Work out the finished part from the listing and answer in its coordinate system (mm). A direction names the side the tool comes from. Coordinates: 2 decimals unless noted, no trailing zeros. Order: outer loops, then holes, each group sorted by start corner. A loop starts at its lowest first (then second) coordinate and runs counter-clockwise, first axis right, second up. Notation, with made-up numbers: (64.25, 39.5) -> (82.25, 39.5) arc R27 ccw to (82.25, 64.5) -> close; hole circle Ø4 at (36.5, 80.5). An arc over 180 degrees is marked (long way). Answer as CSV lines item,"result". Start each with the question number.
Item 1: This flat-tipped pin is pushed along its axis until it touches: pin 1 Ø6.5 at (x, y) = (28.5, 50.6) entering from +Z. Where does it stop, or does it pass through?
Item 2: For a pull along X with two mould halves and no side action, classify faces 3 (the face through (-34.65, -72.09, -3.04)), 4 (the face through (-1, 1, -6)), 5 (the face through (20.1, -45, -3)) as pulls with the +X half, pulls with the -X half, needs draft (parallel to the pull), parting line crosses it, or undercut.
Item 3: Section A-A (x = -15) is taken. Write down the section's boundary in (y, z), then the cut area to 3 significant figures.
Item 4: Which of the six approach directions +Z, -Z, +X, -X, +Y, -Y give full straight-line access (tool end or side, diameter ignored) to faces 1 (the face through (34.49, 72.25, -3.04)), 2 (the face through (-20.1, -45, -3))?
Item 5: Section D-D (y = -44) is taken. Write down the section's boundary in (x, z), then the cut area to 3 significant figures.
Item 6: Section C-C (x = 0) is taken. Write down the section's boundary in (y, z).
Item 7: Straight lines are drawn through the part: L1, parallel to Y at x = 0, z = -3.7; L2, parallel to Y at x = -15, z = -4.4; L3, parallel to X at y = -49, z = -2.8. For each, find the intervals that lie inside material, in ascending order.
Item 8: Section B-B (y = 50.6) is taken. Write down the section's boundary in (x, z).
```python
from build123d import *

# Parameters (mm, degrees)
CROQUIS2_W              = 75
CROQUIS2_H              = 150.2
CROQUIS2_R              = 3.5
CROQUIS2_R_2            = 1.5
CROQUIS2_R_3            = 6.5
CROQUIS2_W_2            = 40.2
CROQUIS2_H_2            = 40.2
SALIENTE_EXTRUIR1_DEPTH = 6
CROQUIS3_R              = 7.5
CORTAR_EXTRUIR1_DEPTH   = 13
REDONDEO1_R             = 10


with BuildPart() as part:
    # Croquis2 → Saliente-Extruir1 (new body)
    with BuildSketch(Plane.XY):
        Rectangle(CROQUIS2_W, CROQUIS2_H)
        with Locations((-28.5, 50.6)):
            Circle(CROQUIS2_R, mode=Mode.SUBTRACT)
        with Locations((28.5, 50.6)):
            Circle(CROQUIS2_R, mode=Mode.SUBTRACT)
        with Locations((0, 66.6)):
            Circle(CROQUIS2_R, mode=Mode.SUBTRACT)
        with Locations((0, -19.9)):
            Circle(CROQUIS2_R_2, mode=Mode.SUBTRACT)
        with Locations((-15, -19.9)):
            Circle(CROQUIS2_R_2, mode=Mode.SUBTRACT)
        with Locations((15, -19.9)):
            Circle(CROQUIS2_R_2, mode=Mode.SUBTRACT)
        with Locations((-15, -70.1)):
            Circle(CROQUIS2_R_2, mode=Mode.SUBTRACT)
        with Locations((0, -70.1)):
            Circle(CROQUIS2_R_2, mode=Mode.SUBTRACT)
        with Locations((15, -70.1)):
            Circle(CROQUIS2_R_2, mode=Mode.SUBTRACT)
        with Locations((0, 50.6)):
            Circle(CROQUIS2_R_3, mode=Mode.SUBTRACT)
        with Locations((0, -45)):
            Rectangle(CROQUIS2_W_2, CROQUIS2_H_2, mode=Mode.SUBTRACT)
    extrude(amount=-SALIENTE_EXTRUIR1_DEPTH)

    # Croquis3 → Cortar-Extruir1 (cut)
    with BuildSketch(Plane.XY):
        with Locations((-28, -26.156897814)):
            Circle(CROQUIS3_R)
    extrude(amount=-CORTAR_EXTRUIR1_DEPTH, mode=Mode.SUBTRACT)

    # Redondeo1
    redondeo1_edges = [part.edges().sort_by_distance(p)[0] for p in [
        (37.5, -75.1, -3),
        (-37.5, -75.1, -3),
        (-37.5, 75.1, -3),
        (37.5, 75.1, -3),
    ]]
    fillet(redondeo1_edges, radius=REDONDEO1_R)


solid = part.part
```
Checked values:
1,pin 1,"passes through"
2,face 3,"pulls with the -X half"
2,face 4,"needs draft"
2,face 5,"undercut"
3,outline,"(-75.1, -6) -> (-71.6, -6) -> (-71.6, 0) -> (-75.1, 0) -> close; (-68.6, -6) -> (-65.1, -6) -> (-65.1, 0) -> (-68.6, 0) -> close; (-24.9, -6) -> (-21.4, -6) -> (-21.4, 0) -> (-24.9, 0) -> close; (-18.4, -6) -> (75.1, -6) -> (75.1, 0) -> (-18.4, 0) -> close"
3,area,"624 mm^2"
4,face 1,"+Z, -Z, +X, +Y"
4,face 2,"+Z, -Z"
5,outline,"(-37.5, -6) -> (-20.1, -6) -> (-20.1, 0) -> (-37.5, 0) -> close; (20.1, -6) -> (37.5, -6) -> (37.5, 0) -> (20.1, 0) -> close"
5,area,"209 mm^2"
6,outline,"(-75.1, -6) -> (-71.6, -6) -> (-71.6, 0) -> (-75.1, 0) -> close; (-68.6, -6) -> (-65.1, -6) -> (-65.1, 0) -> (-68.6, 0) -> close; (-24.9, -6) -> (-21.4, -6) -> (-21.4, 0) -> (-24.9, 0) -> close; (-18.4, -6) -> (44.1, -6) -> (44.1, 0) -> (-18.4, 0) -> close; (57.1, -6) -> (63.1, -6) -> (63.1, 0) -> (57.1, 0) -> close; (70.1, -6) -> (75.1, -6) -> (75.1, 0) -> (70.1, 0) -> close"
7,L1,"y = -75.1 to -71.6, -68.6 to -65.1, -24.9 to -21.4, -18.4 to 44.1, 57.1 to 63.1, 70.1 to 75.1"
7,L2,"y = -75.1 to -71.6, -68.6 to -65.1, -24.9 to -21.4, -18.4 to 75.1"
7,L3,"x = -37.5 to -20.1, 20.1 to 37.5"
8,outline,"(-37.5, -6) -> (-32, -6) -> (-32, 0) -> (-37.5, 0) -> close; (-25, -6) -> (-6.5, -6) -> (-6.5, 0) -> (-25, 0) -> close; (6.5, -6) -> (25, -6) -> (25, 0) -> (6.5, 0) -> close; (32, -6) -> (37.5, -6) -> (37.5, 0) -> (32, 0) -> close"
